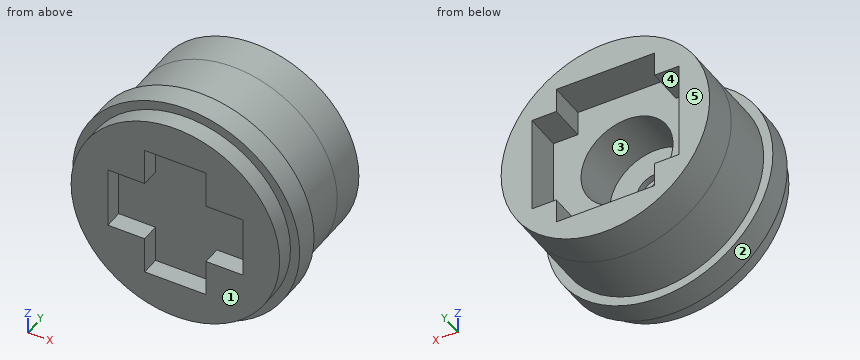
Autodesk Inventor part; units mm, degrees
ref_plane "YZ Plane" through (0, 0, 0) normal (1, 0, 0) x (0, 1, 0)
ref_plane "XZ Plane" through (0, 0, 0) normal (0, 1, 0) x (-1, 0, 0)
ref_plane "XY Plane" through (0, 0, 0) normal (0, 0, 1) x (1, 0, 0)
sketch "Skizze1" plane through (0, 0, 0) normal (0, 1, 0) x (-1, 0, 0)
  circle A0 centre (0, 0) radius 8.5
  line L0 (0, -11.9) -> (0, 11.9)
  line L1 (11.9, 0) -> (-11.9, 0)
  line L2 (6, -6) -> (-6, -6)
  line L3 (-6, -6) -> (-6, 6)
  line L4 (6, 6) -> (6, -6)
  line L5 (6, -6) -> (-6, 6) construction
  line L6 (-6, -6) -> (6, 6) construction
  line L7 (6, 6) -> (-6, 6)
  point P0 (6, -1)
  point P1 (-6, -1)
  dimension "d10" = 12
  dimension "d12" = 17
  dimension "d53" = 12
extrude "Extrusion1" add sketch "Skizze1" along normal blind 6
sketch "Skizze3" plane through (0, 0, 0) normal (0, -1, 0) x (1, 0, 0)
  circle A0 centre (0, 0) radius 8.5
  dimension "d99" = 17
extrude "Extrusion3" add sketch "Skizze3" along normal blind 6
sketch "Skizze9" plane through (0, 6, 0) normal (0, 1, 0) x (1, 0, 0)
  line L0 (-6, 6) -> (6, 6)
  line L1 (6, 6) -> (6, -6)
  line L2 (6, -6) -> (-6, -6)
  line L3 (-6, -6) -> (-6, 6)
  line L4 (-6, 6) -> (6, -6) construction
  line L5 (6, 6) -> (-6, -6) construction
  point P0 (0, 0)
  dimension "d54" = 12
  dimension "d55" = 12
extrude "Extrusion9" cut sketch "Skizze9" against normal blind 6
sketch "Skizze10" plane through (0, 0, 0) normal (0, 1, 0) x (1, 0, 0)
  circle A0 centre (0, 0) radius 3.75
  dimension "d58" = 7.5
extrude "Extrusion10" cut sketch "Skizze10" against normal blind 4
sketch "Skizze12" plane through (0, 6, 0) normal (0, 1, 0) x (1, 0, 0)
  line L0 (-6, 6) -> (-4, 6)
  line L1 (-4, 6) -> (-4, 4)
  line L2 (-4, 4) -> (-6, 4)
  line L3 (-6, 4) -> (-6, 6)
  line L4 (6, 6) -> (6, -6)
  line L5 (6, 6) -> (4, 6)
  line L6 (4, 6) -> (4, 4)
  line L7 (4, 4) -> (6, 4)
  line L8 (6, 4) -> (6, 6)
  line L9 (6, -6) -> (-6, -6)
  line L10 (-6, -6) -> (-4, -6)
  line L11 (-4, -6) -> (-4, -4)
  line L12 (-4, -4) -> (-6, -4)
  line L13 (-6, -4) -> (-6, -6)
  line L14 (6, -6) -> (4, -6)
  line L15 (4, -6) -> (4, -4)
  line L16 (4, -4) -> (6, -4)
  line L17 (6, -4) -> (6, -6)
  point P0 (0, 0)
  dimension "d64" = 2
  dimension "d65" = 2
  dimension "d66" = 2
  dimension "d67" = 2
  dimension "d68" = 2
  dimension "d69" = 2
  dimension "d70" = 2
  dimension "d71" = 2
extrude "Extrusion12" add sketch "Skizze12" against normal up to surface (6 mm away)
sketch "Skizze13" plane through (0, -6, 0) normal (0, -1, 0) x (1, 0, 0)
  line L0 (-2.5, 5.5) -> (2.5, 5.5)
  line L1 (5.5, 2.5) -> (5.5, -2.5)
  line L2 (2.5, -5.5) -> (-2.5, -5.5)
  line L3 (-5.5, -2.5) -> (-5.5, 2.5)
  line L4 (0, 12.6) -> (0, -12.6)
  line L5 (-12.6, 0) -> (12.6, 0)
  line L6 (2.5, 5.5) -> (2.5, 2.5)
  line L7 (2.5, 2.5) -> (5.5, 2.5)
  line L8 (-2.5, 5.5) -> (-2.5, 2.5)
  line L9 (-2.5, 2.5) -> (-5.5, 2.5)
  line L10 (-2.5, -5.5) -> (-2.5, -2.5)
  line L11 (-2.5, -2.5) -> (-5.5, -2.5)
  line L12 (2.5, -5.5) -> (2.5, -2.5)
  line L13 (2.5, -2.5) -> (5.5, -2.5)
  circle A0 centre (0, 0) radius 8.5
  dimension "d76" = 3
  dimension "d77" = 3
  dimension "d78" = 3
  dimension "d79" = 3
  dimension "d80" = 3
  dimension "d81" = 3
  dimension "d82" = 3
  dimension "d83" = 3
  dimension "d84" = 90
  dimension "d85" = 2.5
  dimension "d86" = 2.5
  dimension "d87" = 2.5
  dimension "d88" = 2.5
  dimension "d89" = 90
  dimension "d90" = 17
extrude "Extrusion13" add sketch "Skizze13" along normal blind 2 contours L8 L9 L3 L5 A0 L4 L0 | L4 A0 L5 L1 L7 L6 L0 | A0 L4 L2 L12 L13 L1 L5 | L5 L3 L11 L10 L2 L4 A0
sketch "Skizze14" plane through (0, -4, 0) normal (0, 1, 0) x (1, 0, 0)
  circle A0 centre (0, 0) radius 1.6
  dimension "d93" = 3.2
extrude "Extrusion14" cut sketch "Skizze14" against normal up to surface (2 mm away)
sketch "Skizze15" plane through (0, 6, 0) normal (0, 1, 0) x (1, 0, 0)
  circle A0 centre (0, 0) radius 9
  line L0 (-4, 6) -> (4, 6)
  line L1 (-4, 6) -> (4, 6)
  line L2 (4, 4) -> (6, 4)
  line L3 (4, 6) -> (4, 4)
  line L4 (6, 4) -> (6, -4)
  line L5 (4, 4) -> (6, 4)
  line L6 (6, 4) -> (6, -4)
  line L7 (6, -4) -> (4, -4)
  line L8 (4, -4) -> (4, -6)
  line L9 (4, -4) -> (4, -6)
  line L10 (4, -6) -> (-4, -6)
  line L11 (4, -6) -> (-4, -6)
  line L12 (-4, -4) -> (-4, -6)
  line L13 (-4, -6) -> (-4, -4)
  line L14 (-6, -4) -> (-4, -4)
  line L15 (-4, -4) -> (-6, -4)
  line L16 (-4, 4) -> (-6, 4)
  line L17 (-6, -4) -> (-6, 4)
  line L18 (-6, 4) -> (-4, 4)
  line L19 (-4, 4) -> (-4, 6)
  line L20 (-4, 4) -> (-4, 6)
  dimension "d96" = 18
extrude "Extrusion15" cut sketch "Skizze15" against normal blind 3
ref_plane "Arbeitsebene2" through (0, -6.5, 0) normal (0, -1, 0) x (1, 0, 0)
sketch "Skizze17" plane through (0, -6.5, 0) normal (0, -1, 0) x (1, 0, 0)
  circle A0 centre (0, 0) radius 9.25
  dimension "d102" = 18.5
extrude "Extrusion16" add sketch "Skizze17" against normal blind 2
properties part number "_3D-Druck"
Input: part model. Units: mm. Frame: model coordinates. Face numbers are marked on the shaded views. A direction names the side the tool comes from. Round coordinates to 2 decimals unless told otherwise and drop trailing zeros. Loops run counter-clockwise (first coordinate to the right, second up) from the corner with the lowest first, then second, coordinate; pieces in that order, holes last. Notation, with made-up numbers: M -27,13.5 L 16,13.5 A27 cw 16,39.5 Z; hole C 2,13 d1. An arc over 180 degrees is marked long. Answer in a Markdown table with one row per item. Add a question column.
1. Contact query for flat-ended pins moving along their axis: pin 1 (1.6 mm diameter, centred on y = 2, z = 5, fed in from +X); pin 2 (1.2 mm diameter, centred on y = -7.5, z = -4.5, fed in from -X); pin 3 (1.6 mm diameter, centred on x = -5, y = 1, fed in from +Z). Output: stop coordinate, or through.
2. Set-up query: the marked faces 4 and 5. Return all of +Z, -Z, +X, -X, +Y, -Y with unobstructed straight access to the full face (end or side cutting, diameter ignored); none if empty.
3. Ray query, probe 1 along Z at (x, y) = (0, -2.8); probe 2 along X at (y, z) = (-4.25, 0). Return the intervals inside material, ascending.
4. Mould query, pull axis Z, two halves, no side actions, for the marked faces 1, 2 and 3. Classes: released by +Z, released by -Z, zero draft, split by the parting line, or undercut.
5. Section B-B (z = 4.25). Output: boundary loops of the cut face in (x, y), and give its area (3 significant figures).
6. Section A-A (y = 2). Output: boundary loops of the cut face in (x, z), and give its area (3 significant figures).
7. Section D-D (y = -5.5). Output: boundary loops of the cut face in (x, z).
8. Section C-C (x = 0). Output: boundary loops of the cut face in (y, z), and give its area (3 significant figures).
Values follow:
| question | item | result |
|---|---|---|
| 1 | pin 1 | x = 7.39 |
| 1 | pin 2 | x = -7.55 |
| 1 | pin 3 | z = 7.39 |
| 2 | face 4 | +Y |
| 2 | face 5 | +Z, -Z, +X, -X, +Y |
| 3 | probe 1 | -8.5 to -3.75, 3.75 to 8.5 |
| 3 | probe 2 | -8.5 to -1.6, 1.6 to 8.5 |
| 4 | face 1 | zero draft |
| 4 | face 2 | split by the parting line |
| 4 | face 3 | undercut |
| 5 | outline | M -8.22,-6.5 L -7.36,-6.5 L -7.36,-8 L -2.5,-8 L -2.5,-6.5 L 2.5,-6.5 L 2.5,-8 L 7.36,-8 L 7.36,-6.5 L 8.22,-6.5 L 8.22,-4.5 L 7.36,-4.5 L 7.36,3 L 4,3 L 4,0 L -4,0 L -4,3 L -7.36,3 L -7.36,-4.5 L -8.22,-4.5 Z |
| 5 | area | 134 mm^2 |
| 6 | outline | C 0,0 d17; hole M -6,-4 L -4,-4 L -4,-6 L 4,-6 L 4,-4 L 6,-4 L 6,4 L 4,4 L 4,6 L -4,6 L -4,4 L -6,4 Z |
| 6 | area | 99.0 mm^2 |
| 7 | outline | C 0,0 d18.5 |
| 8 | outline | M -8,-8.5 L -6.5,-8.5 L -6.5,-9.25 L -4.5,-9.25 L -4.5,-8.5 L 3,-8.5 L 3,-6 L 0,-6 L 0,-3.75 L -4,-3.75 L -4,-1.6 L -4.5,-1.6 L -4.5,1.6 L -4,1.6 L -4,3.75 L 0,3.75 L 0,6 L 3,6 L 3,8.5 L -4.5,8.5 L -4.5,9.25 L -6.5,9.25 L -6.5,8.5 L -8,8.5 L -8,5.5 L -6.5,5.5 L -6.5,-5.5 L -8,-5.5 Z |
| 8 | area | 106 mm^2 |
